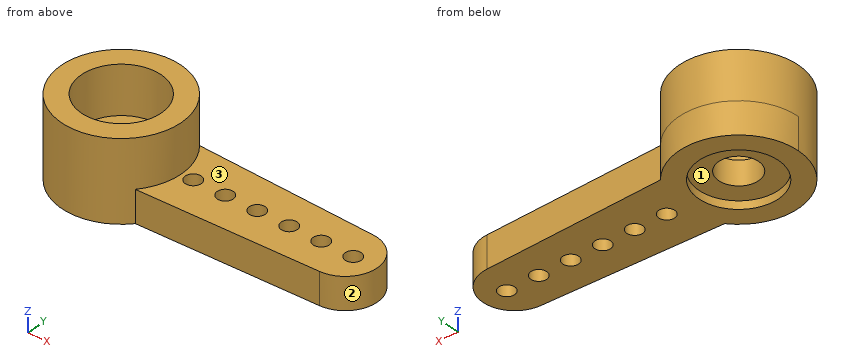
from build123d import *

# Parameters (mm, degrees)
EXTRUDE_3_DEPTH     = 2
EXTRUDE_3_2_DEPTH   = 2
SKETCH_2_R          = 3.75
SKETCH_2_R_2        = 2.5
EXTRUDE_5_DEPTH     = 3
SKETCH_3_R          = 3.75
SKETCH_3_R_2        = 2.5
EXTRUDE_6_DEPTH     = 2
SKETCH_4_R          = 0.5
CUT_EXTRUDE_1_DEPTH = 2
SKETCH_5_R          = 2.5
EXTRUDE_7_DEPTH     = 1
SKETCH_6_R          = 2.5
CUT_EXTRUDE_2_DEPTH = 0.5
SKETCH_7_R          = 1.25
CUT_EXTRUDE_3_DEPTH = 5


with BuildPart() as part:
    # Sketch 1 → Extrude 3 (new body)
    with BuildSketch(Plane.XY):
        with BuildLine():
            ThreePointArc((-0.233236, 2.489096416), (-1.84838984, 1.683286963), (-2.5, 0))
            ThreePointArc((-2.5, 0), (-1.84838984, -1.683286963), (-0.233236, -2.489096416))
            Line((-0.233236, -2.489096416), (0, -2.497361401))
            Line((0, -2.497361401), (0.233236, -2.489096416))
            ThreePointArc((0.233236, -2.489096416), (2.5, 0), (0.233236, 2.489096416))
            Line((0.233236, 2.489096416), (0, 2.497361401))
            Line((0, 2.497361401), (-0.233236, 2.489096416))
        make_face()
    extrude(amount=EXTRUDE_3_DEPTH)



with BuildPart() as body_2:
    # Sketch 1 → Extrude 3 2 (new body)
    with BuildSketch(Plane.XY):
        with BuildLine():
            Line((14.07082784, 1.998745461), (2.88547071, 2.395111434))
            ThreePointArc((2.88547071, 2.395111434), (3.75, 0), (2.88547071, -2.395111434))
            Line((2.88547071, -2.395111434), (14.07082784, -1.998745461))
            ThreePointArc((14.07082784, -1.998745461), (16, 0), (14.07082784, 1.998745461))
        make_face()
    extrude(amount=EXTRUDE_3_2_DEPTH)


with BuildPart() as body_3:
    # Sketch 2 → Extrude 5 (new body)
    with BuildSketch(Plane.XY.offset(2)):
        Circle(SKETCH_2_R)
        Circle(SKETCH_2_R_2, mode=Mode.SUBTRACT)
    extrude(amount=EXTRUDE_5_DEPTH)


with BuildPart() as part_1:
    add(part.part)

    add(body_2.part)  # Extrude 6 merges body 2

    add(body_3.part)  # Extrude 6 merges body 3
    # Sketch 3 → Extrude 6 (add)
    with BuildSketch(Plane(origin=(0, 0, 2), x_dir=(-1, 0, 0), z_dir=(0, 0, -1))):
        Circle(SKETCH_3_R)
        Circle(SKETCH_3_R_2, mode=Mode.SUBTRACT)
    extrude(amount=EXTRUDE_6_DEPTH)

    # Sketch 4 → Cut-Extrude 1 (cut)
    with BuildSketch(Plane(origin=(0, 0, 0), x_dir=(-1, 0, 0), z_dir=(0, 0, -1))):
        with Locations((-14.5, 0)):
            Circle(SKETCH_4_R)
        with Locations((-4.5, 0)):
            Circle(SKETCH_4_R)
        with Locations((-6.5, 0)):
            Circle(SKETCH_4_R)
        with Locations((-8.5, 0)):
            Circle(SKETCH_4_R)
        with Locations((-10.5, 0)):
            Circle(SKETCH_4_R)
        with Locations((-12.5, 0)):
            Circle(SKETCH_4_R)
    extrude(amount=-CUT_EXTRUDE_1_DEPTH, mode=Mode.SUBTRACT)

    # Sketch 5 → Extrude 7 (add)
    with BuildSketch(Plane(origin=(0, 0, 0), x_dir=(-1, 0, 0), z_dir=(0, 0, -1))):
        Circle(SKETCH_5_R)
    extrude(amount=-EXTRUDE_7_DEPTH)

    # Sketch 6 → Cut-Extrude 2 (cut)
    with BuildSketch(Plane(origin=(0, 0, 0), x_dir=(-1, 0, 0), z_dir=(0, 0, -1))):
        Circle(SKETCH_6_R)
    extrude(amount=-CUT_EXTRUDE_2_DEPTH, mode=Mode.SUBTRACT)

    # Sketch 7 → Cut-Extrude 3 (cut)
    with BuildSketch(Plane(origin=(0, 0, 0.5), x_dir=(-1, 0, 0), z_dir=(0, 0, -1))):
        Circle(SKETCH_7_R)
    extrude(amount=-CUT_EXTRUDE_3_DEPTH, mode=Mode.SUBTRACT)


solid = part_1.part
Verification items for the finished model (mm, model axes). Face numbers are marked on the shaded views. Round coordinates to 2 decimals unless told otherwise and drop trailing zeros. Order: outer loops, then holes, each group sorted by start corner. A loop starts at its lowest first (then second) coordinate and runs counter-clockwise, first axis right, second up. Notation, with made-up numbers: (88, 60.5) -> (105, 60.5) arc R20 ccw to (105, 88.5) -> close; hole circle Ø11 at (12, 50.25). An arc over 180 degrees is marked (long way). Put each result on its own line as item: value.
1) Section check B-B (z = 4.55). Record the cut outline in (x, y).
Final values:
outline: circle Ø7.5 at (0, 0); hole circle Ø5 at (0, 0)
2) Depth check by flat-ended pin: pin 1 (2.5 mm diameter, centred on x = 0.5, y = 1, fed in from +Z); pin 2 (3 mm diameter, centred on x = 0, y = 0, fed in from -Z); pin 3 (1.5 mm diameter, centred on x = 0, y = 0, fed in from -Z); pin 4 (2 mm diameter, centred on y = 0.5, z = 2, fed in from -X). Enter the tip coordinate at first touch or a pass-through.
Final values:
pin 1: stops at z = 2
pin 2: stops at z = 0.5
pin 3: passes through
pin 4: stops at x = -3.75
3) Section check A-A (x = 14.5). Record the cut outline in (y, z).
Final values:
outline: (-1.94, 0) -> (-0.5, 0) -> (-0.5, 2) -> (-1.94, 2) -> close; (0.5, 0) -> (1.94, 0) -> (1.94, 2) -> (0.5, 2) -> close
4) Section check C-C (x = 8.5). Record the cut outline in (y, z), then the cut area to 3 significant figures.
Final values:
outline: (-2.2, 0) -> (-0.5, 0) -> (-0.5, 2) -> (-2.2, 2) -> close; (0.5, 0) -> (2.2, 0) -> (2.2, 2) -> (0.5, 2) -> close
area: 6.78 mm^2
5) Material ranges on line 1 (Y direction, x = 0, z = 3.95); line 2 (Z direction, x = 4, y = -2); line 3 (Y direction, x = 1, z = 1), recorded low to high.
Final values:
line 1: y = -3.75 to -2.5, 2.5 to 3.75
line 2: z = 0 to 2
line 3: y = -3.61 to -0.75, 0.75 to 3.61
6) Section check D-D (y = 1.5). Record the cut outline in (x, z), then the cut area to 3 significant figures.
Final values:
outline: (-3.44, 0) -> (-2, 0) -> (-2, 0.5) -> (2, 0.5) -> (2, 0) -> (15.32, 0) -> (15.32, 2) -> (3.44, 2) -> (3.44, 5) -> (2, 5) -> (2, 2) -> (-2, 2) -> (-2, 5) -> (-3.44, 5) -> close
area: 44.1 mm^2
7) Mould release check, pull along Y, two halves, no side actions. Record for the marked faces 1, 2 and 3: +Y half, -Y half, draft (parallel to the pull), parting line (faces both ways), or undercut.
Final values:
face 1: undercut
face 2: parting line
face 3: draft
